Design review of the part built by this model. Coordinates are the model's own, in mm. A direction names the side the tool comes from. Give positions to 0.01 mm unless a question says otherwise; leave off trailing zeros. Write each loop counter-clockwise with the first axis right and the second up, starting at its lowest first coordinate (ties: lowest second). Pieces come first, ordered by that corner, then holes.
```python
from build123d import *

# Parameters (mm, degrees)
SKETCH1_W           = 10.67
SKETCH1_H           = 9.25
BOSS_EXTRUDE1_DEPTH = 4.83
CUT_EXTRUDE1_DEPTH  = 11.67
CUT_EXTRUDE2_DEPTH  = 10.25
CUT_EXTRUDE3_DEPTH  = 11.67
CUT_EXTRUDE4_DEPTH  = 11.67
SKETCH7_R           = 1
CUT_EXTRUDE5_DEPTH  = 3.43
CUT_EXTRUDE5_TAPER  = 3
SKETCH8_R           = 0.5
CUT_EXTRUDE6_DEPTH  = 0.1


with BuildPart() as part:
    # Sketch1 → Boss-Extrude1 (new body)
    with BuildSketch(Plane(origin=(0, 0, 0), x_dir=(1, 0, 0), z_dir=(0, 1, 0))):
        Rectangle(SKETCH1_W, SKETCH1_H)
    extrude(amount=BOSS_EXTRUDE1_DEPTH)

    # Sketch3 → Cut-Extrude1 (cut, through all)
    with BuildSketch(Plane(origin=(5.335, 0, 0), x_dir=(0, 0, -1), z_dir=(1, 0, 0))):
        Polygon((4.625, 4.83), (4.225, 4.83), (4.625, 1.39), align=None)
    extrude(amount=-CUT_EXTRUDE1_DEPTH, mode=Mode.SUBTRACT)

    # Sketch4 → Cut-Extrude2 (cut, through all)
    with BuildSketch(Plane.XY.offset(4.625)):
        Polygon((5.335, 4.83), (5.135, 4.83), (5.335, 3.66), align=None)
    cut_extrude2 = extrude(amount=-CUT_EXTRUDE2_DEPTH, mode=Mode.SUBTRACT)

    # Mirror1: Cut-Extrude2 across plane
    add(cut_extrude2.mirror(Plane(origin=(0, 0, 0), x_dir=(0, 0, 1), z_dir=(1, 0, 0))), mode=Mode.SUBTRACT)

    # Sketch5 → Cut-Extrude3 (cut, through all)
    with BuildSketch(Plane.ZY.offset(5.335)):
        Polygon((4.425, 4.83), (4.625, 4.83), (4.625, 3.66), align=None)
    extrude(amount=-CUT_EXTRUDE3_DEPTH, mode=Mode.SUBTRACT)

    # Sketch6 → Cut-Extrude4 (cut, through all)
    with BuildSketch(Plane.ZY.offset(5.335)):
        Polygon((4.625, 0), (4.625, 3.05), (4.425, 0), align=None)
    extrude(amount=-CUT_EXTRUDE4_DEPTH, mode=Mode.SUBTRACT)

    # Sketch7 → Cut-Extrude5 (cut)
    with BuildSketch(Plane(origin=(0, 4.83, 0), x_dir=(1, 0, 0), z_dir=(0, 1, 0))):
        with Locations((-5.335, 0)):
            Circle(SKETCH7_R)
    cut_extrude5 = extrude(amount=-CUT_EXTRUDE5_DEPTH, taper=CUT_EXTRUDE5_TAPER, mode=Mode.SUBTRACT)

    # Mirror2: Cut-Extrude5 across plane
    add(cut_extrude5.mirror(Plane(origin=(0, 0, 0), x_dir=(0, 0, 1), z_dir=(1, 0, 0))), mode=Mode.SUBTRACT)

    # Sketch8 → Cut-Extrude6 (cut)
    with BuildSketch(Plane(origin=(0, 4.83, 0), x_dir=(1, 0, 0), z_dir=(0, 1, 0))):
        with Locations((-4.135, -3.425)):
            Circle(SKETCH8_R)
    extrude(amount=-CUT_EXTRUDE6_DEPTH, mode=Mode.SUBTRACT)


solid = part.part
```
(1) Consider section A-A, the plane z = 0. Give the boundary of the cut face in (x, y) (3 decimals), then the cut area to 3 significant figures.
Resolved:
outline: (-5.335, 0) - (5.335, 0) - (5.335, 1.4) - (4.515, 1.4) - (4.335, 4.83) - (-4.335, 4.83) - (-4.515, 1.4) - (-5.335, 1.4) - close
area: 45.3 mm2
(2) Tool access review of faces 5 (the face through (-4.1, 4.73, 3.4)), 6 (the face through (5, 1.4, 0)), 7 (the face through (5.335, 1, 0)): name each direction out of +Z, -Z, +X, -X, +Y, -Y from which nothing blocks a thin tool from reaching the whole face with its end or side.
Resolved:
face 5: +Y
face 6: +X, +Y
face 7: +Z, -Z, +X, +Y, -Y
(3) Clearance check with flat-ended pins moving along their axes: P1, Ø1, axis at x = -3, y = 3, coming from the -Z side; P2, Ø0.5, axis at x = -4, z = 3.5, coming from the +Y side. State where each tip first meets the part, or that it passes through.
Resolved:
P1: stops at z = -4.5
P2: stops at y = 4.73
(4) To check wall thickness, follow L1, parallel to Z at x = 4.5, y = 3.45 (3 decimals); L2, parallel to Z at x = 1.75, y = 3.8; L3, parallel to Z at x = 4, y = 2.35. State the ranges of each line that lie inside material, in increasing order.
Resolved:
L1: z = -4.385 to -0.404, 0.404 to 4.625
L2: z = -4.34 to 4.6
L3: z = -4.51 to 4.58
(5) Mouldability with a two-part tool opening along Z and no side actions: class faces 1 (the face through (-4.426, 3.091, 0.02)), 2 (the face through (-5, 1.4, 0)), 3 (the face through (5.234, 4.253, -2.626)), 4 (the face through (0, 1, -4.625)) as pulls with the +Z half, pulls with the -Z half, needs draft (parallel to the pull), parting line crosses it, or undercut.
Resolved:
face 1: undercut
face 2: undercut
face 3: needs draft
face 4: pulls with the -Z half
(6) Consider section B-B, the plane x = -2.5. Give the boundary of the cut face in (y, z) (3 decimals), then the cut area to 3 significant figures.
Resolved:
outline: (0, -4.625) - (1.39, -4.625) - (4.83, -4.225) - (4.83, 4.425) - (3.66, 4.625) - (3.05, 4.625) - (0, 4.425) - close
area: 43.6 mm2
